Here's how the part is built. I have some questions about the finished solid (model axes, mm). Face numbers are marked on the shaded views. A direction names the side the tool comes from. Coordinates: 2 decimals unless noted, no trailing zeros. Write each loop counter-clockwise with the first axis right and the second up, starting at its lowest first coordinate (ties: lowest second). Pieces come first, ordered by that corner, then holes. Notation, with made-up numbers: (36.25, 15) -> (66.25, 15) arc R8 cw to (66.25, 29) -> close; hole circle Ø4 at (-10, -29.75). An arc over 180 degrees is marked (long way). Put each result on its own line as item: value.
Solid Edge part; units mm, degrees
sketch "Sketch1" plane through (0, 0, 0) normal (0, 0, 1) x (1, 0, 0)
  line L0 (0, 10) -> (50, 10)
  line L1 (50, 10) -> (50, 20)
  line L2 (50, 20) -> (47, 20)
  line L3 (47, 20) -> (47, 45)
  line L4 (47, 45) -> (32, 45)
  line L5 (32, 45) -> (32, 23)
  line L6 (32, 23) -> (29, 23)
  line L7 (29, 23) -> (29, 20)
  line L8 (29, 20) -> (3, 20)
  line L9 (3, 20) -> (3, 18)
  line L10 (3, 18) -> (1.5, 18)
  line L11 (1.5, 18) -> (1.5, 20)
  line L12 (1.5, 20) -> (0, 20)
  line L13 (0, 20) -> (0, 10)
  dimension "D1" = 50
  dimension "D2" = 47
  dimension "D3" = 47
  dimension "D4" = 32
  dimension "D5" = 29
  dimension "D6" = 1.5
  dimension "D7" = 29
  dimension "D8" = 50
  dimension "D9" = 3
  dimension "D10" = 3
revolve "RevolvedProtrusion1" add sketch "Sketch1" angle 360 about axis through (57, 0, 0) along (-1, 0, 0)
sketch "Sketch2" plane through (47, 0, 0) normal (1, 0, 0) x (0, 1, 0)
  line L0 (179.2581, -202.8725) -> (30, -202.8725)
  line L1 (30, -202.8725) -> (30, 202.8725)
  line L2 (30, 202.8725) -> (179.2581, 202.8725)
  line L3 (179.2581, 202.8725) -> (179.2581, -202.8725)
  line L4 (-30, -200.4946) -> (-139.3849, -200.4946)
  line L5 (-139.3849, -200.4946) -> (-139.3849, 200.4946)
  line L6 (-139.3849, 200.4946) -> (-30, 200.4946)
  line L7 (-30, 200.4946) -> (-30, -200.4946)
extrude "Cutout1" cut sketch "Sketch2" against normal blind 2932.3571
sketch "Sketch3" plane through (0, 0, 0) normal (-1, 0, 0) x (0, -1, 0)
  line L0 (-2.5, 7.35) -> (2.5, 7.35)
  line L1 (2.5, 7.35) -> (2.5, 12.65)
  line L2 (2.5, 12.65) -> (-2.5, 12.65)
  line L3 (-2.5, 12.65) -> (-2.5, 7.35)
extrude "ExtrudedProtrusion_2" add sketch "Sketch3" against normal blind 35
sketch "Sketch4" plane through (0, 0, 0) normal (-1, 0, 0) x (0, -1, 0)
  circle A0 centre (0, 0) radius 20
extrude "ExtrudedProtrusion_3" add sketch "Sketch4" against normal blind 3
sketch "Sketch5" plane through (0, 0, 0) normal (-1, 0, 0) x (0, -1, 0)
  circle A0 centre (0, 0) radius 4
extrude "ExtrudedCutout_2" cut sketch "Sketch5" along normal mid plane 90.6479
properties material "Aluminum, 6061-T6"
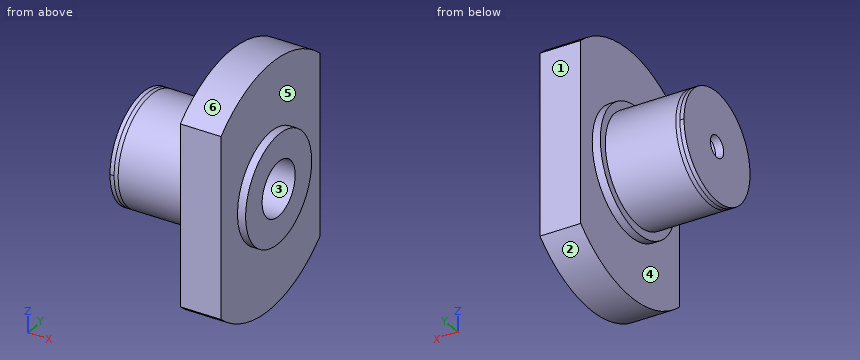
Item 1: If we mould it in two halves opening along Z, with no side actions, what happens to the marked faces 1, 2 and 3? For each: released by +Z, released by -Z, zero draft, split by the parting line, or undercut.
Output:
face 1: zero draft
face 2: released by -Z
face 3: undercut
Item 2: Imagine slicing it at B-B on x = 24.5. Write out the boundary of the cut face in (y, z).
Output:
outline: circle Ø40 at (0, 0); hole (-2.5, 7.35) -> (-2.5, 9.68) arc R10 ccw (long way) to (2.5, 9.68) -> (2.5, 7.35) -> close
Item 3: For P1, Ø12, axis at y = 0, z = 0, coming from the +X side; P2, Ø2, axis at y = 7.5, z = -27.5, coming from the -X side; P3, Ø6, axis at x = 22.5, z = -20, coming from the -Y side, each with a flat end and sliding along its axis, tell me the tip position at first contact or that it passes through.
Output:
P1: stops at x = 3
P2: stops at x = 32
P3: stops at y = -10.54
Item 4: Imagine slicing it at D-D on x = 30. Write out the boundary of the cut face in (y, z), then the cut area to 3 significant figures.
Output:
outline: circle Ø46 at (0, 0); hole (-2.5, 7.35) -> (-2.5, 9.68) arc R10 ccw (long way) to (2.5, 9.68) -> (2.5, 7.35) -> close
area: 1,360 mm²
Item 5: Which directions (+Z, -Z, +X, -X, +Y, -Y) give clear straight access to the entire face, cutting with the end or side of a thin tool? Please do the marked faces 4, 5 and 6.
Output:
face 4: -X
face 5: +X
face 6: +Z, +X, -X
Item 6: Imagine slicing it at C-C on z = 13. Write out the boundary of the cut face in (x, y).
Output:
outline: (0, -15.2) -> (29, -15.2) -> (29, -18.97) -> (32, -18.97) -> (32, -30) -> (47, -30) -> (47, -15.2) -> (50, -15.2) -> (50, 15.2) -> (47, 15.2) -> (47, 30) -> (32, 30) -> (32, 18.97) -> (29, 18.97) -> (29, 15.2) -> (0, 15.2) -> close
Item 7: Please list where these lines run through material, in increasing order: line 1 along Z through (x, y) = (28.5, 0); line 2 along Z through (x, y) = (40.5, 0); line 3 along X through (y, z) = (16, -23). Write a range as from..to.
Output:
line 1: z = -20..-10, 7.35..20
line 2: z = -45..-10, 10..45
line 3: x = 32..47
Item 8: Imagine slicing it at A-A on y = 0. Write out the boundary of the cut face in (x, z), then the cut area to 3 significant figures.
Output:
outline: (0, -20) -> (29, -20) -> (29, -23) -> (32, -23) -> (32, -45) -> (47, -45) -> (47, -20) -> (50, -20) -> (50, -10) -> (3, -10) -> (3, -4) -> (0, -4) -> close; (0, 4) -> (3, 4) -> (3, 7.35) -> (35, 7.35) -> (35, 10) -> (50, 10) -> (50, 20) -> (47, 20) -> (47, 45) -> (32, 45) -> (32, 23) -> (29, 23) -> (29, 20) -> (0, 20) -> close
area: 1,890 mm²
